from build123d import *

# Parameters (mm, degrees)
SKETCH2_W                     = 12.7
SKETCH2_H                     = 84
BOSS_EXTRUDE1_DEPTH           = 12.7
SKETCH5_W                     = 12.7
SKETCH5_H                     = 25
BOSS_EXTRUDE2_DEPTH           = 5
CBORE_FOR_M4_SHCS1_AT_2_COUNT = 2
CBORE_FOR_M4_SHCS1_AT_2_PITCH = 15
CHAMFER1_SIZE                 = 5
SKETCH6_W                     = 41.3
SKETCH6_H                     = 12.7
CUT_EXTRUDE1_DEPTH            = 48.313634399
SKETCH7_W                     = 12.7
SKETCH7_H                     = 12.7
BOSS_EXTRUDE3_DEPTH           = 49.17
SKETCH9_W                     = 12.7
SKETCH9_H                     = 25.1
BOSS_EXTRUDE4_DEPTH           = 13.7
CBORE_FOR_M5_SHCS2_AT_2_COUNT = 2
CBORE_FOR_M5_SHCS2_AT_2_PITCH = 15


with BuildPart() as part:
    # Sketch2 → Boss-Extrude1 (new body)
    with BuildSketch(Plane(origin=(0, 0, 0), x_dir=(1, 0, 0), z_dir=(0, 1, 0))):
        Rectangle(SKETCH2_W, SKETCH2_H)
    extrude(amount=BOSS_EXTRUDE1_DEPTH)

    # Sketch5 → Boss-Extrude2 (add)
    with BuildSketch(Plane(origin=(0, 12.7, 0), x_dir=(1, 0, 0), z_dir=(0, 1, 0))):
        with Locations((0, 29.5)):
            Rectangle(SKETCH5_W, SKETCH5_H)
    extrude(amount=BOSS_EXTRUDE2_DEPTH)

    # Sketch4 → CBORE for M4 SHCS1 (revolve, cut)
    with BuildSketch(Plane(origin=(0, 0, -37), x_dir=(0, 0, -1), z_dir=(1, 0, 0))):
        Polygon((0, 0), (0, 17.7), (2.4, 17.7), (2.4, 4), (4, 4), (4, 0.020977491), (4.025, 0), align=None)
    cbore_for_m4_shcs1 = revolve(axis=Axis((0, -6.35, -37), (0, 1, 0)), mode=Mode.SUBTRACT)

    # CBORE for M4 SHCS1 at 2: CBORE for M4 SHCS1 ×2
    with Locations(*[(0, 0, i * CBORE_FOR_M4_SHCS1_AT_2_PITCH) for i in range(1, CBORE_FOR_M4_SHCS1_AT_2_COUNT)]):
        add(cbore_for_m4_shcs1, mode=Mode.SUBTRACT)

    # Chamfer1
    chamfer1_edges = [part.edges().sort_by_distance(p)[0] for p in [
        (0, 12.7, -17),
    ]]
    chamfer(chamfer1_edges, length=CHAMFER1_SIZE - 0.0001)  # a hair under: the kernel refuses the full size

    # Sketch6 → Cut-Extrude1 (cut, through all)
    with BuildSketch(Plane(origin=(6.35, 0, 0), x_dir=(0, 0, -1), z_dir=(1, 0, 0))):
        with Locations((-21.35, 6.35)):
            Rectangle(SKETCH6_W, SKETCH6_H)
    extrude(amount=-CUT_EXTRUDE1_DEPTH, mode=Mode.SUBTRACT)

    # Sketch7 → Boss-Extrude3 (add)
    with BuildSketch(Plane(origin=(0, 0, 0), x_dir=(-1, 0, 0), z_dir=(0, -1, 0))):
        with Locations((0, 5.65)):
            Rectangle(SKETCH7_W, SKETCH7_H)
    extrude(amount=BOSS_EXTRUDE3_DEPTH)

    # Sketch9 → Boss-Extrude4 (add)
    with BuildSketch(Plane(origin=(-6.35, 0, 0), x_dir=(0, 0, -1), z_dir=(1, 0, 0))):
        with Locations((5.65, -36.62)):
            Rectangle(SKETCH9_W, SKETCH9_H)
    extrude(amount=-BOSS_EXTRUDE4_DEPTH)

    # Sketch14 → CBORE for M5 SHCS2 (revolve, cut)
    with BuildSketch(Plane(origin=(-13.7, -29.12, 0.7), x_dir=(0, -1, 0), z_dir=(1, 0, 0))):
        Polygon((0, 0), (0, 42.7), (2.75, 42.7), (2.75, 5), (5, 5), (5, 0.025), (5.025, 0), align=None)
    cbore_for_m5_shcs2 = revolve(axis=Axis((-13.7, -29.12, 7.05), (0, 0, -1)), mode=Mode.SUBTRACT)

    # CBORE for M5 SHCS2 at 2: CBORE for M5 SHCS2 ×2
    with Locations(*[(0, -i * CBORE_FOR_M5_SHCS2_AT_2_PITCH, 0) for i in range(1, CBORE_FOR_M5_SHCS2_AT_2_COUNT)]):
        add(cbore_for_m5_shcs2, mode=Mode.SUBTRACT)


solid = part.part
CAD build for the part. Positions are in the model's coordinates, mm. A direction names the side the tool comes from. Coordinates: 2 decimals unless noted, no trailing zeros. Order: outer loops, then holes, each group sorted by start corner. A loop starts at its lowest first (then second) coordinate and runs counter-clockwise, first axis right, second up.
Item 1: Two-plate mould, pull along X, no slides. Class faces 4 (the face through (2, 4, -35)), 5 (the face through (-4, -30, -12)), 6 (the face through (-20.05, -36, -6)): +X half, -X half, draft (parallel to the pull), parting line (faces both ways), or undercut.
Check sheet entries:
face 4: undercut
face 5: draft
face 6: -X half
Item 2: Drill centre lines: L1, parallel to Y at x = -13.7, z = -9.5; L2, parallel to X at y = -29.12, z = -8; L3, parallel to X at y = 1.55, z = -22. Where is each one in solid material? Low to high.
Check sheet entries:
L1: y = -49.17 to -46.87, -41.37 to -31.87, -26.37 to -24.07
L2: x = -20.05 to -16.45, -10.95 to 6.35
L3: x = -6.35 to -4, 4 to 6.35
Item 3: Band-saw the part on B-B on y = -44.12. List the corners of the cut face in (x, z) (3 decimals).
Check sheet entries:
outline: (-20.05, -12) - (-16.45, -12) - (-16.45, -4.3) - (-18.7, -4.3) - (-18.7, 0.675) - (-18.725, 0.7) - (-20.05, 0.7) - close; (-10.95, -12) - (6.35, -12) - (6.35, 0.7) - (-8.675, 0.7) - (-8.7, 0.675) - (-8.7, -4.3) - (-10.95, -4.3) - close
Item 4: 3-axis set-ups, long thin cutter, end or side, ignore diameter. For faces 1 (the face through (0, 0, -27)), 2 (the face through (-18.657, -43.469, -1.778)), 3 (the face through (-13, -24.07, -6)): which of +Z, -Z, +X, -X, +Y, -Y reach the whole face in a straight line?
Check sheet entries:
face 1: -Z, +X, -X, -Y
face 2: +Z
face 3: +Z, -Z, -X, +Y
Item 5: Band-saw the part on D-D on z = -3. List the corners of the cut face in (x, y).
Check sheet entries:
outline: (-20.05, -49.17) - (6.35, -49.17) - (6.35, 12.7) - (-6.35, 12.7) - (-6.35, -24.07) - (-20.05, -24.07) - close; hole circle Ø10 at (-13.7, -44.12); hole circle Ø10 at (-13.7, -29.12)
Item 6: Band-saw the part on A-A on z = -37. List the corners of the cut face in (x, y) (3 decimals).
Check sheet entries:
outline: (-6.35, 0) - (-4.025, 0) - (-4, 0.021) - (-4, 4) - (-2.4, 4) - (-2.4, 17.7) - (-6.35, 17.7) - close; (2.4, 4) - (4, 4) - (4, 0.021) - (4.025, 0) - (6.35, 0) - (6.35, 17.7) - (2.4, 17.7) - close
Item 7: Pin check, flat tips, straight feed: pin 1 Ø9 at (x, z) = (0, -21) entering from -Y; pin 2 Ø2 at (x, z) = (-5.5, -10.5) entering from +Y; pin 3 Ø3 at (x, y) = (-12, -30) entering from +Z. Stop position of each tip, or through.
Check sheet entries:
pin 1: stops at y = 0
pin 2: stops at y = 12.7
pin 3: stops at z = -4.3
Item 8: Band-saw the part on C-C on x = 0. Give the number of separate pieces and of enclosed holes in the cut face, plus the area to 3 significant figures.
Check sheet entries:
separate pieces: 3
enclosed holes: 0
area: 1,110 mm2
